For this review, take the finished solid that the model builds, in its own axes (mm). A direction names the side the tool comes from. Round coordinates to 2 decimals unless told otherwise and drop trailing zeros. Order: outer loops, then holes, each group sorted by start corner. A loop starts at its lowest first (then second) coordinate and runs counter-clockwise, first axis right, second up. Notation, with made-up numbers: (81.5, 86.25) -> (126.5, 86.25) arc R21 ccw to (126.5, 93.25) -> close; hole circle Ø11 at (48, 13). An arc over 180 degrees is marked (long way). Use a Markdown table: item, result. Add a question column.
1) Draft analysis for pull direction Z (two halves, no side actions). For faces 3 (the face through (1, 0, -1)), 4 (the face through (15.02, 2.71, 47.69)), 5 (the face through (-11.753, 4.268, -3.613)), state which applies: pulls with the +Z half, pulls with the -Z half, needs draft (parallel to the pull), parting line crosses it, or undercut.
2) Consider section A-A (y = 3.9). State the section outline as (x, z) points, plus the area to 3 significant figures.
3) Consider section D-D (x = -23.5). State the section outline as (y, z) points, plus the area to 3 significant figures.
4) Consider section B-B (x = 0). State the section outline as (y, z) points, plus the area to 3 significant figures.
5) Wall thickness on line 1 along Z through (x, y) = (-46, 2.6); line 2 along Z through (x, y) = (3, 3.95); line 3 along Z through (x, y) = (-4, 3.05): over which ranges is each line inside the solid? List them lowest first. Write a range as [from, to].
6) Machinability: for faces 1 (the face through (1, 5.5, 10)), 2 (the face through (0, 3, 0)), which of the approach directions +Z, -Z, +X, -X, +Y, -Y give a long, thin tool a straight path to every point of the face, cutting with its end or side? Answer none if there is none.
7) Consider section C-C (z = 0). State the section outline as (x, y) points.
8) Clearance check with flat-ended pins moving along their axes: P1, Ø12, axis at x = 33, z = 28.5, coming from the -Y side; P2, Ø2, axis at y = 3.5, z = 1, coming from the +X side; P3, Ø0.8, axis at y = 4, z = 0.5, coming from the -X side; P4, Ø3, axis at x = 26, y = 1, coming from the -Z side. State where each tip first meets the part, or that it passes through.
```python
from build123d import *

# Parameters (mm, degrees)
SKETCH1_R           = 50
BOSS_EXTRUDE1_DEPTH = 5.5
CUT_EXTRUDE1_DEPTH  = 2.5


with BuildPart() as part:
    # Sketch1 → Boss-Extrude1 (new body)
    with BuildSketch(Plane(origin=(0, 0, 0), x_dir=(1, 0, 0), z_dir=(0, 1, 0))):
        with Locations(Location((0, 0, 0), (0, 0, 270))):
            Circle(SKETCH1_R)
    extrude(amount=BOSS_EXTRUDE1_DEPTH)

    # Sketch2 → Cut-Extrude1 (cut)
    with BuildSketch(Plane(origin=(0, 5.5, 0), x_dir=(1, 0, 0), z_dir=(0, 1, 0))):
        with BuildLine():
            Line((-4.043822449, -4.5), (-19.25, -2.75))
            Line((-19.25, -2.75), (-19.25, 2.75))
            Line((-19.25, 2.75), (-4.043822449, 4.5))
            ThreePointArc((-4.043822449, 4.5), (0, 6.05), (4.043822449, 4.5))
            Line((4.043822449, 4.5), (19.25, 2.75))
            Line((19.25, 2.75), (19.25, -2.75))
            Line((19.25, -2.75), (4.043822449, -4.5))
            ThreePointArc((4.043822449, -4.5), (0, -6.05), (-4.043822449, -4.5))
        make_face()
    extrude(amount=-CUT_EXTRUDE1_DEPTH, mode=Mode.SUBTRACT)


solid = part.part
```
Results list:
| question | item | result |
|---|---|---|
| 1 | face 3 | needs draft |
| 1 | face 4 | parting line crosses it |
| 1 | face 5 | undercut |
| 2 | outline | circle Ø100 at (0, 0); hole (-19.25, -2.75) -> (-4.04, -4.5) arc R6.05 ccw to (4.04, -4.5) -> (19.25, -2.75) -> (19.25, 2.75) -> (4.04, 4.5) arc R6.05 ccw to (-4.04, 4.5) -> (-19.25, 2.75) -> close |
| 2 | area | 7,540 mm2 |
| 3 | outline | (0, -44.13) -> (5.5, -44.13) -> (5.5, 44.13) -> (0, 44.13) -> close |
| 3 | area | 485 mm2 |
| 4 | outline | (0, -50) -> (5.5, -50) -> (5.5, -6.05) -> (3, -6.05) -> (3, 6.05) -> (5.5, 6.05) -> (5.5, 50) -> (0, 50) -> close |
| 4 | area | 520 mm2 |
| 5 | line 1 | [-19.6, 19.6] |
| 5 | line 2 | [-49.91, -5.25], [5.25, 49.91] |
| 5 | line 3 | [-49.84, -4.54], [4.54, 49.84] |
| 6 | face 1 | +Z, -Z, +X, -X, +Y |
| 6 | face 2 | +Y |
| 7 | outline | (-50, 0) -> (50, 0) -> (50, 5.5) -> (19.25, 5.5) -> (19.25, 3) -> (-19.25, 3) -> (-19.25, 5.5) -> (-50, 5.5) -> close |
| 8 | P1 | y = 0 |
| 8 | P2 | x = 50 |
| 8 | P3 | x = -50 |
| 8 | P4 | z = -43.59 |
